Part print with two shaded views. Sizes in mm from the minimum x, y, z corner. Round coordinates to 2 decimals unless told otherwise and drop trailing zeros. Loops run counter-clockwise (first coordinate to the right, second up) from the corner with the lowest first, then second, coordinate; pieces in that order, holes last. Notation, with made-up numbers: (55, 26) - (109, 26) arc R16 cw to (109, 48) - close; hole circle Ø10 at (65.5, 50.5). An arc over 180 degrees is marked (long way). One line per question, with ' | ' between items.
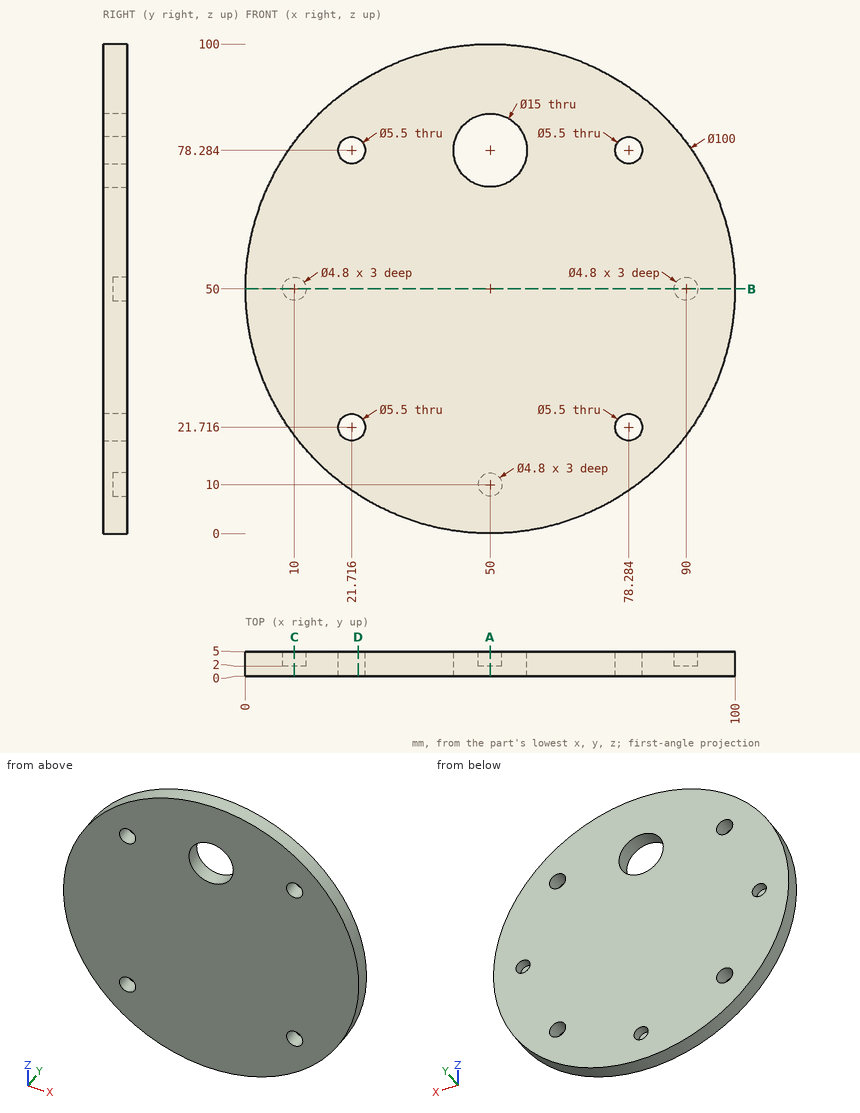
(1) Cut at D-D, the plane x = 23. Write the cut outline in (y, z).
Results found:
outline: (0, 7.92) - (5, 7.92) - (5, 19.28) - (0, 19.28) - close; (0, 24.15) - (5, 24.15) - (5, 75.85) - (0, 75.85) - close; (0, 80.72) - (5, 80.72) - (5, 92.08) - (0, 92.08) - close
(2) Cut at C-C, the plane x = 10. Write the cut outline in (y, z), then the cut area to 3 significant figures.
Results found:
outline: (0, 20) - (5, 20) - (5, 47.6) - (2, 47.6) - (2, 52.4) - (5, 52.4) - (5, 80) - (0, 80) - close | area: 286 mm²
(3) Probe L1, parallel to X at y = 3.8, z = 48 (1 decimal); L2, parallel to X at y = 0.3, z = 20.5; L3, parallel to Z at x = 78.5, y = 3.7 (1 decimal). List the from-to ranges inside material, lowest first.
Results found:
L1: x = 0 to 8.7, 11.3 to 88.7, 91.3 to 100 | L2: x = 9.63 to 19.25, 24.18 to 75.82, 80.75 to 90.37 | L3: z = 8.9 to 19, 24.5 to 75.5, 81 to 91.1
(4) Cut at A-A, the plane x = 50. Write the cut outline in (y, z).
Results found:
outline: (0, 0) - (5, 0) - (5, 7.6) - (2, 7.6) - (2, 12.4) - (5, 12.4) - (5, 70.78) - (0, 70.78) - close; (0, 85.78) - (5, 85.78) - (5, 100) - (0, 100) - close
(5) Drop flat-ended pins along their axis: P1, Ø7.5, axis at x = 10, z = 50, coming from the -Y side; P2, Ø2.5, axis at x = 9, z = 49.5, coming from the +Y side; P3, Ø3, axis at y = 2.5, z = 85, coming from the +X side; P4, Ø3.5, axis at x = 21.72, z = 78.28, coming from the -Y side. Give the stop position or say it passes through.
Results found:
P1: stops at y = 0 | P2: stops at y = 2 | P3: stops at x = 87.12 | P4: passes through
(6) Cut at B-B, the plane z = 50. Write the cut outline in (x, y).
Results found:
outline: (0, 0) - (100, 0) - (100, 5) - (92.4, 5) - (92.4, 2) - (87.6, 2) - (87.6, 5) - (12.4, 5) - (12.4, 2) - (7.6, 2) - (7.6, 5) - (0, 5) - close
